Work out the finished part from the listing and answer in its coordinate system (mm). Coordinates: 2 decimals unless noted, no trailing zeros. Loops run counter-clockwise (first coordinate to the right, second up) from the corner with the lowest first, then second, coordinate; pieces in that order, holes last. Notation, with made-up numbers: (-39, 56.5) - (13, 56.5) arc R23 cw to (13, 78.5) - close; hole circle Ø2 at (-3.5, 89). An arc over 180 degrees is marked (long way). Write each question's results on one line, items separated by ' | '. Start each with the question number.
1. A cutting plane is placed at A-A on y = 1. Determine the outline of the cut face in (x, z), then the cut area to 3 significant figures.
2. This flat-tipped pin is pushed along its axis until it touches: P1, Ø1.5, axis at x = -30, y = 1, coming from the -Z side. Where does it stop, or does it pass through?
3. Find the intervals of material crossed by line 1 along Z through (x, y) = (-26, -0.75); line 2 along X through (y, z) = (-1, 17.5); line 3 along X through (y, z) = (0, -18), in increasing order. Write a range as [from, to].
4. A cutting plane is placed at B-B on x = -31. Determine the outline of the cut face in (y, z) (3 decimals), then the cut area to 3 significant figures.
5. A cutting plane is placed at C-C on z = 17. Determine the outline of the cut face in (x, y) (3 decimals).
from build123d import *

# Parameters (mm, degrees)
F1_DEPTH = 3.175


with BuildPart() as f1:
    # F0 (on Front) → F1 (new body, symmetric)
    with BuildSketch(Plane.XZ):
        with BuildLine():
            Line((-25.4, -25.4), (25.4, -25.4))
            ThreePointArc((25.4, -25.4), (34.3802561211, -21.6802561211), (38.1, -12.7))
            Line((38.1, -12.7), (38.1, 12.7))
            ThreePointArc((38.1, 12.7), (34.3802561211, 21.6802561211), (25.4, 25.4))
            Line((25.4, 25.4), (-25.4, 25.4))
            ThreePointArc((-25.4, 25.4), (-34.3802561211, 21.6802561211), (-38.1, 12.7))
            Line((-38.1, 12.7), (-38.1, -12.7))
            ThreePointArc((-38.1, -12.7), (-34.3802561211, -21.6802561211), (-25.4, -25.4))
        make_face()
    extrude(amount=F1_DEPTH, both=True)


solid = f1.part
Values:
1) outline: (-38.1, -12.7) arc R12.7 ccw to (-25.4, -25.4) - (25.4, -25.4) arc R12.7 ccw to (38.1, -12.7) - (38.1, 12.7) arc R12.7 ccw to (25.4, 25.4) - (-25.4, 25.4) arc R12.7 ccw to (-38.1, 12.7) - close | area: 3,730 mm^2
2) P1: z = -24.8
3) line 1: [-25.39, 25.39] | line 2: [-37.16, 37.16] | line 3: [-36.94, 36.94]
4) outline: (-3.175, -24.099) - (3.175, -24.099) - (3.175, 24.099) - (-3.175, 24.099) - close | area: 306 mm^2
5) outline: (-37.35, -3.175) - (37.35, -3.175) - (37.35, 3.175) - (-37.35, 3.175) - close
